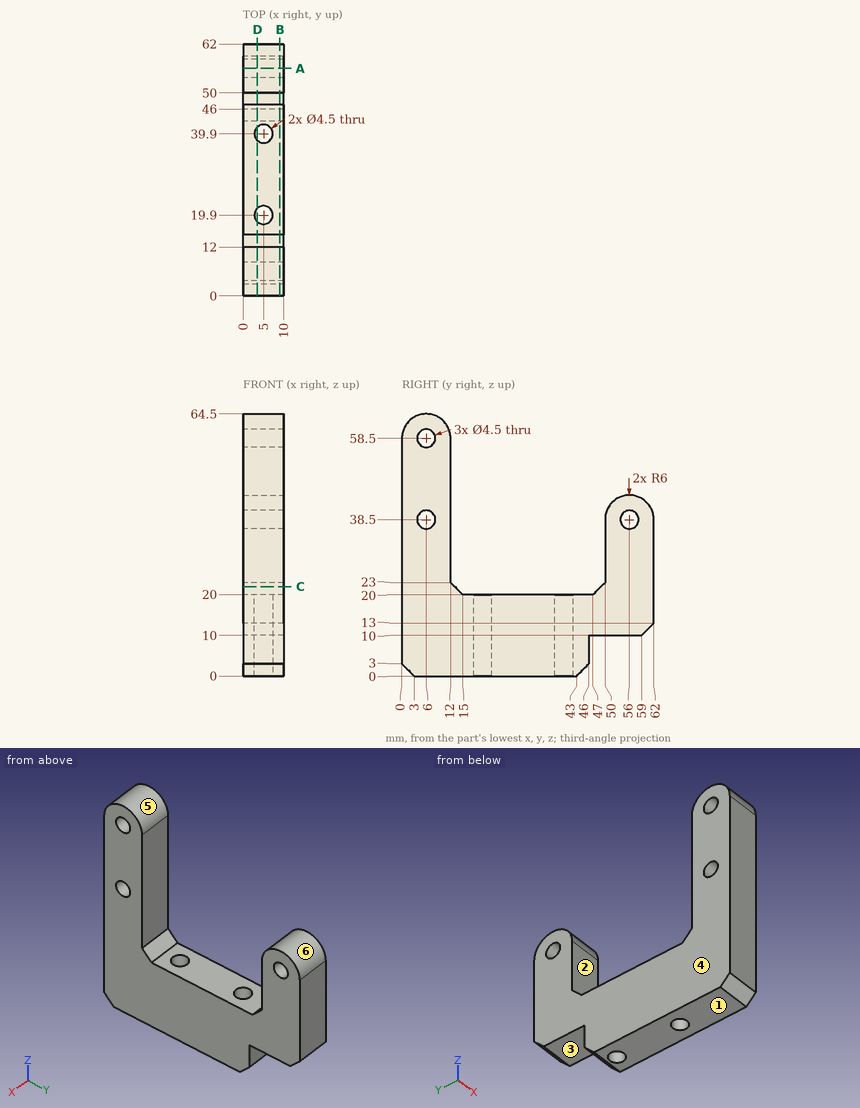
Source: three-view drawing plus pictorial views. Frame: mm from the lowest corner of the part. A direction names the side the tool comes from. Round coordinates to 2 decimals unless told otherwise and drop trailing zeros. Order: outer loops, then holes, each group sorted by start corner. A loop starts at its lowest first (then second) coordinate and runs counter-clockwise, first axis right, second up. Notation, with made-up numbers: (-13.75, 67.5) - (38.25, 67.5) arc R26 ccw to (38.25, 97.5) - close; hole circle Ø2 at (37, -19.5). An arc over 180 degrees is marked (long way). Write each question's results on one line, items separated by ' | '.
Item 1: Reachability of the marked faces 1, 2 and 3 from +Z, -Z, +X, -X, +Y, -Y: full face, straight path, thin tool, end or side. Return the list, or none.
Completed:
face 1: -Z, +X, -X, +Y, -Y | face 2: +Z, +X, -X | face 3: -Z, +X, -X, +Y
Item 2: Mould query, pull axis Y, two halves, no side actions, for the marked faces 4, 5 and 6. Classes: pulls with the +Y half, pulls with the -Y half, needs draft (parallel to the pull), parting line crosses it, or undercut.
Completed:
face 4: needs draft | face 5: parting line crosses it | face 6: undercut
Item 3: Material intervals for line 1 along Y through (x, z) = (6.75, 34); line 2 along Z through (x, y) = (3.5, 8); line 3 along X through (y, z) = (19.9, 6.25), sorted ascending. Write a range as [from, to].
Completed:
line 1: [0, 12], [50, 62] | line 2: [0, 37.47], [39.53, 57.47], [59.53, 64.16] | line 3: [0, 2.75], [7.25, 10]
Item 4: Section C-C, the plane z = 22. Return the cut outline in (x, y).
Completed:
outline: (0, 0) - (10, 0) - (10, 13) - (0, 13) - close; (0, 49) - (10, 49) - (10, 62) - (0, 62) - close
Item 5: Section D-D, the plane x = 3.5. Return the cut outline in (y, z).
Completed:
outline: (0, 3) - (3, 0) - (18.22, 0) - (18.22, 20) - (15, 20) - (12, 23) - (12, 58.5) arc R6 ccw to (0, 58.5) - close; (21.58, 0) - (38.22, 0) - (38.22, 20) - (21.58, 20) - close; (41.58, 0) - (43, 0) - (46, 3) - (46, 10) - (59, 10) - (62, 13) - (62, 38.5) arc R6 ccw to (50, 38.5) - (50, 23) - (47, 20) - (41.58, 20) - close; hole circle Ø4.5 at (6, 38.5); hole circle Ø4.5 at (6, 58.5); hole circle Ø4.5 at (56, 38.5)
Item 6: Section B-B, the plane x = 9. Return the cut outline in (y, z).
Completed:
outline: (0, 3) - (3, 0) - (43, 0) - (46, 3) - (46, 10) - (59, 10) - (62, 13) - (62, 38.5) arc R6 ccw to (50, 38.5) - (50, 23) - (47, 20) - (15, 20) - (12, 23) - (12, 58.5) arc R6 ccw to (0, 58.5) - close; hole circle Ø4.5 at (6, 38.5); hole circle Ø4.5 at (6, 58.5); hole circle Ø4.5 at (56, 38.5)
Item 7: First-contact query: pin 1 Ø2.5 at (y, z) = (56, 38.5) entering from -X; pin 2 Ø3 at (x, y) = (8.5, 37) entering from +Z; pin 3 Ø4 at (x, y) = (6, 49) entering from +Z; pin 4 Ø5 at (x, y) = (7.5, 53.5) entering from -Z. Flat tips, straight axial feed; report the tip coordinate or a pass-through.
Completed:
pin 1: through | pin 2: z = 20 | pin 3: z = 41.82 | pin 4: z = 10
Item 8: Section A-A, the plane y = 56. Return the cut outline in (x, z), and give its area (3 significant figures).
Completed:
outline: (0, 10) - (10, 10) - (10, 36.25) - (0, 36.25) - close; (0, 40.75) - (10, 40.75) - (10, 44.5) - (0, 44.5) - close | area: 300 mm^2
